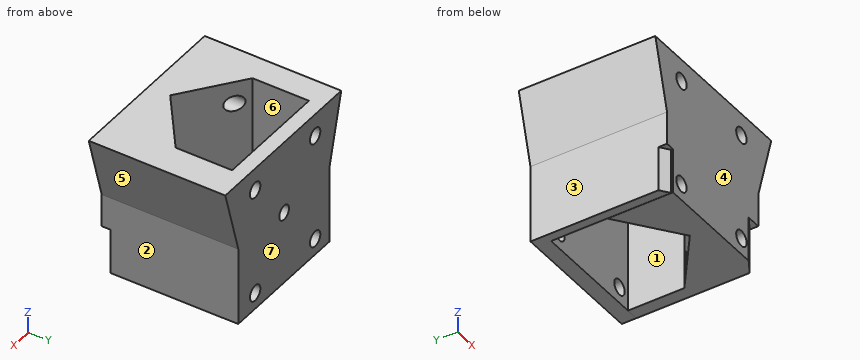
Autodesk Inventor part; units mm, degrees
ref_plane "РабПлоскость2" through (0, 0, -5) normal (0, 0, -1) x (-1, 0, 0)
ref_plane "РабПлоскость4" through (5.0978, 14.8061, 0.0339) normal (0, 1, 0) x (-1, 0, 0)
ref_plane "РабПлоскость5" through (5.0978, 4.5741, 0.0339) normal (0, 1, 0) x (-1, 0, 0)
ref_plane "РабПлоскость2" through (0, 0, -5) normal (0, 0, -1) x (-1, 0, 0)
sketch "Эскиз1" plane through (0, 0, -5) normal (0, 0, -1) x (-1, 0, 0)
  line L0 (-19.4986, 4.5741) -> (-16.2986, 4.5741)
  line L1 (-1.0261, 4.5741) -> (2.1739, 4.5741)
  line L2 (-25.5748, 4.5741) -> (-23.7748, 4.5741)
  line L3 (5.4196, 4.5741) -> (7.2196, 4.5741)
  line L4 (-20.4986, 4.5741) -> (3.1739, 4.5741)
  line L5 (3.1739, 4.5741) -> (3.1739, 9.0001)
  line L6 (3.1739, 9.0001) -> (-20.4986, 9.0001)
  line L7 (-20.4986, 9.0001) -> (-20.4986, 4.5741)
  line L8 (-38.6624, 4.5741) -> (21.3376, 4.5741)
  point P0 (0, 0)
  point P1 (-20.4986, 6.7871)
  point P2 (3.1739, 6.7871)
  dimension "d0" = 1
  dimension "d1" = 1
  dimension "d3" = 4.426
extrude "Выдавливание1" add sketch "Эскиз1" against normal blind 30
ref_plane "РабПлоскость3" through (5.0978, 4.5741, 0.0339) normal (0, 1, 0) x (-1, 0, 0)
sketch "Эскиз3" plane through (0, 0, 25) normal (0, 0, 1) x (1, 0, 0)
  line L0 (20.4986, 4.5741) -> (20.4986, 9.0001)
  line L1 (20.4986, 9.0001) -> (20.4986, 18.0001)
  line L2 (20.4986, 18.0001) -> (8.6624, 9.0001)
  line L3 (20.4986, 9.0001) -> (-3.1739, 9.0001)
  line L4 (-3.1739, 9.0001) -> (-3.1739, 4.5741)
  line L5 (-3.1739, 18.0001) -> (-3.1739, 9.0001)
  line L6 (-3.1739, 18.0001) -> (8.6624, 9.0001)
  point P0 (0, 0)
  dimension "d8" = 9
  dimension "d9" = 9
extrude "Выдавливание3" add sketch "Эскиз3" against normal up to surface (30 mm away)
ref_plane "РабПлоскость4" through (5.0978, 14.8061, 0.0339) normal (0, 1, 0) x (-1, 0, 0)
sketch "Эскиз2" plane through (5.0978, 4.5741, 0.0339) normal (0, 1, 0) x (-1, 0, 0)
  circle A0 centre (-31.4768, 2.1354) radius 0.9
  circle A1 centre (23.5157, 1.4536) radius 0.9
  circle A2 centre (-19.4778, 1.9866) radius 0.9
  circle A3 centre (-19.5769, -6.0128) radius 0.9
  circle A4 centre (23.4165, -6.5458) radius 0.9
  circle A5 centre (11.5166, 1.6023) radius 0.9
  circle A6 centre (11.4174, -6.3971) radius 0.9
  circle A7 centre (-31.576, -5.864) radius 0.9
  circle A8 centre (-12.8008, -1.6339) radius 1.6
  circle A9 centre (5.6717, -1.6339) radius 1.6
  circle A10 centre (-12.8008, 20.3661) radius 1.6
  circle A11 centre (5.6717, 20.3661) radius 1.6
  arc A12 (11.4355, 36.4061) -> (11.4355, 44.3661) centre (11.4355, 40.3861) ccw
  line L0 (11.4355, 44.3661) -> (-18.5645, 44.3661)
  arc A13 (-18.5645, 44.3661) -> (-18.5645, 36.4061) centre (-18.5645, 40.3861) ccw
  line L1 (-18.5645, 36.4061) -> (11.4355, 36.4061)
  line L2 (-33.5645, -20.6339) -> (-33.5645, 49.3661)
  line L3 (-33.5645, 49.3661) -> (26.4355, 49.3661)
  line L4 (26.4355, 49.3661) -> (26.4355, -20.6339)
  line L5 (26.4355, -20.6339) -> (-33.5645, -20.6339)
  point P0 (5.0978, -0.0339)
extrude "дырки" cut sketch "Эскиз2" along normal through all contours A8 | A9 | A10 | A11
sketch "Эскиз4" plane through (5.0978, 14.8061, 0.0339) normal (0, 1, 0) x (-1, 0, 0)
  circle A0 centre (-12.8008, -1.6339) radius 1.6
  circle A1 centre (-12.8008, 20.3661) radius 1.6
  line L0 (-15.4008, -5.0339) -> (-3.5645, -5.0339)
  line L1 (-3.5645, 24.9661) -> (-3.5645, -5.0339)
  line L2 (-15.4008, 24.9661) -> (-3.5645, 24.9661)
  line L3 (-15.4008, 24.9661) -> (-15.4008, -5.0339)
  circle A2 centre (5.6717, -1.6339) radius 1.6
  circle A3 centre (5.6717, 20.3661) radius 1.6
  line L4 (-3.5645, -5.0339) -> (8.2717, -5.0339)
  line L5 (8.2717, 24.9661) -> (8.2717, -5.0339)
  line L6 (-3.5645, 24.9661) -> (8.2717, 24.9661)
  line L7 (-3.5645, 24.9661) -> (-3.5645, -5.0339)
  circle A4 centre (-12.8008, 20.3661) radius 2.1992
  circle A5 centre (5.6717, 20.3661) radius 2.3283
  circle A6 centre (-12.8008, -1.6339) radius 2.1992
  circle A7 centre (5.6717, -1.6339) radius 2.3283
  point P0 (5.0978, -0.0339)
ref_plane "РабПлоскость5" through (5.0978, 4.5741, 0.0339) normal (0, 1, 0) x (-1, 0, 0)
sketch "Эскиз5" plane through (5.0978, 4.5741, 0.0339) normal (0, 1, 0) x (-1, 0, 0)
  line L0 (-15.4008, -5.0339) -> (-3.5645, -5.0339)
  line L1 (-3.5645, 24.9661) -> (-3.5645, -5.0339)
  line L2 (-15.4008, 24.9661) -> (-3.5645, 24.9661)
  line L3 (-15.4008, 24.9661) -> (-15.4008, -5.0339)
  line L4 (-3.5645, -5.0339) -> (8.2717, -5.0339)
  line L5 (8.2717, 24.9661) -> (8.2717, -5.0339)
  line L6 (-3.5645, 24.9661) -> (8.2717, 24.9661)
  line L7 (-3.5645, 24.9661) -> (-3.5645, -5.0339)
  line L8 (-15.4008, -5.0339) -> (-18, -5.0339)
  line L9 (-18, -5.0339) -> (-18, 24.9661)
  line L10 (-18, 24.9661) -> (-15.4008, 24.9661)
  line L11 (-15.4008, 24.9661) -> (-15.4008, -5.0339)
  line L12 (8.2717, 24.9661) -> (10.1117, 24.9661)
  line L13 (10.1117, 24.9661) -> (10.1117, -5)
  line L14 (10.1117, -5) -> (8.2717, -5)
  line L15 (8.2717, -5) -> (8.2717, 24.9661)
  line L16 (10.1117, 11) -> (13.7176, 11)
  line L17 (13.7176, 11) -> (13.7176, 24.9661)
  line L18 (13.7176, 24.9661) -> (10.1117, 24.9661)
  line L19 (10.1117, 24.9661) -> (10.1117, 11)
  line L20 (-18, 11) -> (-22, 11)
  line L21 (-22, 11) -> (-22, 24.9661)
  line L22 (-22, 24.9661) -> (-18, 24.9661)
  line L23 (-18, 24.9661) -> (-18, 11)
  line L24 (-22, 24.9661) -> (-18, 11)
  line L25 (10.1117, 11) -> (13.7176, 24.9661)
  point P0 (5.0978, -0.0339)
  point P1 (-15.4008, 24.9661)
  point P2 (8.2717, -5)
  dimension "d22" = 1.84
extrude "Выдавливание5" add sketch "Эскиз5" along normal blind 25 contours L8 L9 L10 L3 | L9 L24 L22 | L12 L13 L14 L5 | L18 L25 L13
sketch "Эскиз6" plane through (5.0978, 29.5741, 0.0339) normal (0, 1, 0) x (1, 0, 0)
  line L0 (15.4008, 5.0339) -> (15.4008, -24.9661)
  line L1 (15.4008, -24.9661) -> (22, -24.9661)
  line L2 (22, -24.9661) -> (18, -11)
  line L3 (18, -11) -> (18, 5.0339)
  line L4 (18, 5.0339) -> (15.4008, 5.0339)
  line L5 (-13.7176, -24.9661) -> (-8.2717, -24.9661)
  line L6 (-8.2717, -24.9661) -> (-8.2717, 5)
  line L7 (-8.2717, 5) -> (-10.1117, 5)
  line L8 (-10.1117, 5) -> (-10.1117, -11)
  line L9 (-10.1117, -11) -> (-13.7176, -24.9661)
  line L10 (15.4008, -24.9661) -> (22, -24.9661)
  line L11 (15.4008, -24.9661) -> (-8.2717, -24.9661)
  line L12 (18, -11) -> (18, 5.0339)
  line L13 (18, 5) -> (-10.1117, 5)
  circle A0 centre (3.8883, -9.9661) radius 1.5
  point P0 (-5.0978, 0.0339)
  dimension "d17" = 15
  dimension "d18" = 14
  dimension "d19" = 3
extrude "Выдавливание6" add sketch "Эскиз6" along normal blind 3 contours L13 L3 L2 L1 L0 | L0 L11 L6 L13 | L6 L5 L9 L8 L7
sketch "Эскиз7" plane through (5.0978, 32.5741, 0.0339) normal (0, 1, 0) x (1, 0, 0)
  circle A0 centre (12.8008, -20.3661) radius 1.6
  circle A1 centre (-5.6717, -20.3661) radius 1.6
  circle A2 centre (-5.6717, 1.6339) radius 1.6
  circle A3 centre (12.8008, 1.6339) radius 1.6
  point P0 (-5.0978, 0.0339)
extrude "Выдавливание7" cut sketch "Эскиз7" against normal through all
sketch "Эскиз9" plane through (0, 0, -5) normal (0, 0, -1) x (-1, 0, 0)
  line L0 (-23.0978, 4.5741) -> (-23.0978, 29.5741)
  line L1 (-23.0978, 29.5741) -> (-20.4986, 29.5741)
  line L2 (-20.4986, 29.5741) -> (-20.4986, 18.0001)
  line L3 (-20.4986, 18.0001) -> (-8.6624, 9.0001)
  line L4 (-8.6624, 9.0001) -> (3.1739, 18.0001)
  line L5 (3.1739, 18.0001) -> (3.1739, 4.5741)
  line L6 (3.1739, 4.5741) -> (-23.0978, 4.5741)
  line L7 (-23.0978, 6.3376) -> (-20.1479, 4.5741)
  line L8 (5.0139, 4.5741) -> (5.0139, 32.5741)
  line L9 (5.0139, 6.3376) -> (2.6946, 4.5741)
  line L10 (3.1739, 4.5741) -> (5.0139, 4.5741)
  point P0 (0, 0)
  point P1 (3.1739, 4.9385)
extrude "Выдавливание9" cut sketch "Эскиз9" against normal blind 9.25 contours L0 L7 L6 | L5 L9 L8 L10
properties part number "крепеж_маркера"
Geometry check sheet. Reference: the model listing, model coordinates, mm. Face numbers are marked on the shaded views. A direction names the side the tool comes from. Give positions to 0.01 mm unless a question says otherwise; leave off trailing zeros. Write each loop counter-clockwise with the first axis right and the second up, starting at its lowest first coordinate (ties: lowest second). Pieces come first, ordered by that corner, then holes.
1) Cross-section at C-C (y = 7.75). Count the separate pieces of the cut face and the enclosed holes in it, plus the area to 3 significant figures.
Values follow:
separate pieces: 1
enclosed holes: 4
area: 864 mm2
2) Thickness scan on line 1 (X direction, y = 31.05, z = 10); line 2 (X direction, y = 30.75, z = -1.6); line 3 (X direction, y = 27.5, z = 6.5). Record the ranges inside material, lowest first.
Values follow:
line 1: x = -5.01 to 7.49, 10.49 to 23.1
line 2: x = -5.01 to -2.17, 1.03 to 16.3, 19.5 to 23.1
line 3: x = -5.01 to -3.17, 20.5 to 23.1
3) Cross-section at D-D (x = 7). Record the boundary of the cut face in (y, z).
Values follow:
outline: (4.57, -5) - (10.26, -5) - (10.26, 25) - (4.57, 25) - close; (29.57, -4.97) - (32.57, -4.97) - (32.57, 25) - (29.57, 25) - close
4) Go/stop test with flat-tipped pins: pin 1 Ø8 at (y, z) = (23, 8.5) entering from +X; pin 2 Ø8 at (y, z) = (21, 6) entering from -X; pin 3 Ø8.5 at (x, y) = (13.5, 25.5) entering from -Z; pin 4 Ø2.5 at (x, z) = (17.9, -1.6) entering from +Y. Record where each tip stops, or that it passes through.
Values follow:
pin 1: stops at x = 23.52
pin 2: stops at x = -5.01
pin 3: stops at z = -4.97
pin 4: passes through
5) Cross-section at A-A (y = 30.5). Record the boundary of the cut face in (x, z).
Values follow:
outline: (-8.62, 25) - (-5.01, 11.03) - (-5.01, -4.97) - (23.1, -4.97) - (23.1, 11.03) - (27.1, 25) - close; hole circle Ø3.2 at (-0.57, -1.6); hole circle Ø3.2 at (-0.57, 20.4); hole circle Ø3 at (8.99, 10); hole circle Ø3.2 at (17.9, -1.6); hole circle Ø3.2 at (17.9, 20.4)
6) Cross-section at B-B (z = 2). Record the boundary of the cut face in (x, y), plus the area to 3 significant figures.
Values follow:
outline: (-5.01, 6.34) - (-3.17, 4.94) - (-3.17, 4.57) - (20.15, 4.57) - (23.1, 6.34) - (23.1, 32.57) - (-5.01, 32.57) - close; hole (-3.17, 18) - (8.66, 9) - (20.5, 18) - (20.5, 29.57) - (-3.17, 29.57) - close
area: 402 mm2
7) Release check for a two-part mould opening along Y. For the marked faces 5, 6 and 7 record: released by +Y, released by -Y, zero draft, split by the parting line, or undercut.
Values follow:
face 5: zero draft
face 6: undercut
face 7: released by +Y
8) Set-up check for the marked faces 1, 2, 3 and 4: record each of +Z, -Z, +X, -X, +Y, -Y from which the full face is reachable in a straight line by a thin tool's end or side.
Values follow:
face 1: +Z, -Z
face 2: -Z, +X, +Y, -Y
face 3: -Z, -X, +Y, -Y
face 4: +Z, -Z, +X, -X, -Y
